```python
from build123d import *

# Parameters (mm, degrees)
EXTRUDE_1_DEPTH     = 46.5
SKETCH_4_OUTSIDE_W  = 66.66
SKETCH_4_OUTSIDE_H  = 64.16
CUT_EXTRUDE_1_DEPTH = 50
SHELL_START         = 6
SHELL_1_DEPTH       = 40.5
SHELL_START_2       = 8.5
SHELL_1_2_DEPTH     = 38
SHELL_START_3       = -22.293752824
SHELL_1_3_DEPTH     = 44.587505647
SKETCH_5_R          = 20.5
EXTRUDE_3_DEPTH     = 8
FILLET_1_R          = 5
SKETCH_4_8_R        = 3
CUT_EXTRUDE_3_DEPTH = 48
FILLET_3_R          = 3
SKETCH_8_W          = 65
SKETCH_8_H          = 50
SKETCH_8_R          = 3.25
EXTRUDE_4_DEPTH     = 8


with BuildPart() as part:
    # 草图1 → 凸台-拉伸1 (new body)
    with BuildSketch(Plane.XY):
        with BuildLine():
            ThreePointArc((35.945795724, -14), (32.1298187, -14.493507683), (28.564936874, -15.941557419))
            Line((28.564936874, -15.941557419), (25.184577361, -17.852195404))
            ThreePointArc((25.184577361, -17.852195404), (17.819425425, -19.7937446), (10.450223542, -17.867624161))
            ThreePointArc((10.450223542, -17.867624161), (0, 0), (10.450223542, 17.867624161))
            ThreePointArc((10.450223542, 17.867624161), (17.819425425, 19.7937446), (25.184577361, 17.852195404))
            Line((25.184577361, 17.852195404), (28.564936874, 15.941557419))
            ThreePointArc((28.564936874, 15.941557419), (32.1298187, 14.493507683), (35.945795724, 14))
            Line((35.945795724, 14), (49, 14))
            Line((49, 14), (49, -14))
            Line((49, -14), (35.945795724, -14))
        make_face()
    extrude(amount=EXTRUDE_1_DEPTH)

    # 草图4 outside → 切除-拉伸1 (cut, symmetric)
    with BuildSketch(Plane.XZ.offset(14)):
        with Locations((24.5, 23.25)):
            Rectangle(SKETCH_4_OUTSIDE_W, SKETCH_4_OUTSIDE_H)
        with BuildLine():
            Line((49, 36.813688531), (44, 8.5))
            Line((44, 8.5), (0, 8.5))
            Line((0, 8.5), (0, 9.114014501))
            Line((0, 9.114014501), (5, 9.114014501))
            ThreePointArc((5, 9.114014501), (9.499546785, 10.183500589), (13.036653031, 13.163198754))
            Line((13.036653031, 13.163198754), (35.472510226, 43.46311181))
            ThreePointArc((35.472510226, 43.46311181), (38.125339912, 45.697885434), (41.5, 46.5))
            Line((41.5, 46.5), (49, 46.5))
            Line((49, 46.5), (49, 36.813688531))
        make_face(mode=Mode.SUBTRACT)
    extrude(amount=CUT_EXTRUDE_1_DEPTH, both=True, mode=Mode.SUBTRACT)

    # 抽壳1: read off the stored shape, not the designer's step
    # 抽壳1 outline → 抽壳1 (add)
    with BuildSketch(Plane.XY.offset(SHELL_START)):
        with BuildLine():
            Line((49, -16.5), (49, 16.5))
            Line((49, 16.5), (35.945796372, 16.5))
            ThreePointArc((35.945796372, 16.5), (32.765815184, 16.91125632), (29.795080015, 18.117964516))
            Line((29.795080015, 18.117964516), (26.414720503, 20.028602501))
            ThreePointArc((26.414720503, 20.028602501), (17.822043244, 22.293743229), (9.224641048, 20.046602717))
            ThreePointArc((9.224641048, 20.046602717), (-2.5, 3.232e-06), (9.224641048, -20.046602717))
            ThreePointArc((9.224641048, -20.046602717), (17.822043244, -22.293743229), (26.414720503, -20.028602501))
            Line((26.414720503, -20.028602501), (29.795080015, -18.117964516))
            ThreePointArc((29.795080015, -18.117964516), (32.765815184, -16.91125632), (35.945796372, -16.5))
            Line((35.945796372, -16.5), (49, -16.5))
        make_face()
    extrude(amount=SHELL_1_DEPTH)

    # Shell 1 2 outline → Shell 1 2 (cut)
    with BuildSketch(Plane.XY.offset(SHELL_START_2)):
        with BuildLine():
            Line((25.184577361, -17.852195404), (28.564936874, -15.941557419))
            ThreePointArc((28.564936874, -15.941557419), (32.129818701, -14.493507683), (35.945795724, -14))
            Line((35.945795724, -14), (49, -14))
            Line((49, -14), (49, 14))
            Line((49, 14), (35.945795724, 14))
            ThreePointArc((35.945795724, 14), (32.129818701, 14.493507683), (28.564936874, 15.941557419))
            Line((28.564936874, 15.941557419), (25.184577361, 17.852195404))
            ThreePointArc((25.184577361, 17.852195404), (17.819425424, 19.7937446), (10.450223542, 17.867624161))
            ThreePointArc((10.450223542, 17.867624161), (0, 0), (10.450223542, -17.867624161))
            ThreePointArc((10.450223542, -17.867624161), (17.819425424, -19.7937446), (25.184577361, -17.852195404))
        make_face()
    extrude(amount=SHELL_1_2_DEPTH, mode=Mode.SUBTRACT)

    # Shell 1 3 outline → Shell 1 3 (cut)
    with BuildSketch(Plane(origin=(0, 0, 0), x_dir=(1, 0, 0), z_dir=(0, 1, 0)).offset(SHELL_START_3)):
        with BuildLine():
            Line((-4, -46.5), (41.5, -46.5))
            ThreePointArc((41.5, -46.5), (38.125339907, -45.697885432), (35.47251022, -43.463111802))
            Line((35.47251022, -43.463111802), (13.036653031, -13.163198754))
            ThreePointArc((13.036653031, -13.163198754), (9.499546673, -10.183500533), (4.999999751, -9.114014501))
            Line((4.999999751, -9.114014501), (-4, -9.114014501))
            Line((-4, -9.114014501), (-4, -46.5))
        make_face()
        Polygon((49, -36.813688531), (49, -6), (43.558517429, -6), align=None)
    extrude(amount=SHELL_1_3_DEPTH, mode=Mode.SUBTRACT)

    # 草图5 → 凸台-拉伸3 (add)
    with BuildSketch(Plane(origin=(0, 0, 6), x_dir=(-1, 0, 0), z_dir=(0, 0, -1))):
        with Locations(Location((-18, 0, 0), (0, 0, 359.999469823))):
            Circle(SKETCH_5_R)
    extrude(amount=EXTRUDE_3_DEPTH)

    # 圆角1
    fillet_1_edges = [part.edges().sort_by_distance(p)[0] for p in [
        (38.499999999, 0.000189693, -2),
    ]]
    fillet(fillet_1_edges, radius=FILLET_1_R)

    # 草图4<8> → 切除-拉伸3 (cut, symmetric)
    with BuildSketch(Plane.XZ.offset(14)):
        with Locations(Location((41.5, 39, 0), (0, 0, 270))):
            Circle(SKETCH_4_8_R)
    extrude(amount=CUT_EXTRUDE_3_DEPTH, both=True, mode=Mode.SUBTRACT)

    # 圆角3
    fillet_3_edges = [part.edges().sort_by_distance(p)[0] for p in [
        (49, -15.25, 46.5),
        (49, 15.25, 46.5),
    ]]
    fillet(fillet_3_edges, radius=FILLET_3_R)

    # 草图8 → 凸台-拉伸4 (add)
    with BuildSketch(Plane(origin=(0, 0, -2), x_dir=(-1, 0, 0), z_dir=(0, 0, -1))):
        with Locations((-18, 0)):
            Rectangle(SKETCH_8_W, SKETCH_8_H)
        with Locations((6.5, 18.846153846)):
            Circle(SKETCH_8_R, mode=Mode.SUBTRACT)
        with Locations((6.5, -18.846153846)):
            Circle(SKETCH_8_R, mode=Mode.SUBTRACT)
        with Locations((-42.5, -18.846153846)):
            Circle(SKETCH_8_R, mode=Mode.SUBTRACT)
        with Locations((-42.5, 18.846153846)):
            Circle(SKETCH_8_R, mode=Mode.SUBTRACT)
    extrude(amount=EXTRUDE_4_DEPTH)


solid = part.part
```
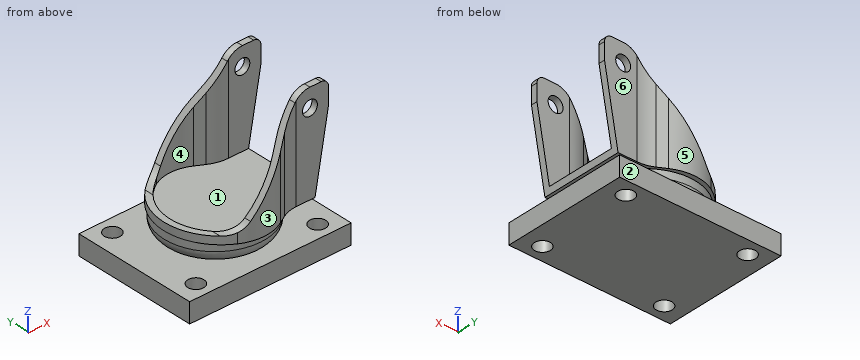
The listing builds one solid part. Answer for the finished solid, in the listing's coordinates (mm). Face numbers are marked on the shaded views. A direction names the side the tool comes from. Coordinates: 2 decimals unless noted, no trailing zeros. Loops run counter-clockwise (first coordinate to the right, second up) from the corner with the lowest first, then second, coordinate; pieces in that order, holes last. Notation, with made-up numbers: (59, 10.25) -> (79, 10.25) arc R21 cw to (79, 41.25) -> close; hole circle Ø7 at (46.25, 48). An arc over 180 degrees is marked (long way). Return JSON: item names as keys, results as strings. Group by question number.
(1) Find the intervals of material crossed by probe 1 along Y at (x, z) = (42.5, -7.75); probe 2 along Y at (x, z) = (44.5, 17); probe 3 along X at (y, z) = (20, -5.5), in increasing order. Write a range as from..to.
(2) A cutting plane is placed at A-A on x = -6.5. Write down the section's boundary in (y, z).
(3) Given pin 1 Ø14.5 at (x, z) = (40, 22) entering from +Y; pin 2 Ø12 at (x, z) = (41, 28.5) entering from -Y; pin 3 Ø2 at (y, z) = (15.5, 40.5) entering from +X; pin 4 Ø5 at (x, z) = (41.5, 39) entering from +Y, each flat-ended and moving along its own axis, determine where each tip first touches the part or whether it passes through.
(4) Which of the six approach directions +Z, -Z, +X, -X, +Y, -Y give full straight-line access (tool end or side, diameter ignored) to the marked faces 4, 5 and 6?
(5) Determine the mould class of the marked faces 1, 2 and 3 for opening direction Y: released by +Y, released by -Y, zero draft, split by the parting line, or undercut.
(6) A cutting plane is placed at B-B on z = 27. Write down the section's boundary in (x, y).
The answers:
{
 "1": {"probe 1": "y = -25..-22.1, -15.6..15.6, 22.1..25", "probe 2": "y = -16.5..-14, 14..16.5", "probe 3": "x = -14.5..-9.54, -3.46..39.46, 45.54..50.5"},
 "2": {"outline": "(-25, -10) -> (-22.1, -10) -> (-22.1, -2) -> (-25, -2) -> close; (-15.6, -10) -> (15.6, -10) -> (15.6, -2) -> (-15.6, -2) -> close; (22.1, -10) -> (25, -10) -> (25, -2) -> (22.1, -2) -> close"},
 "3": {"pin 1": "stops at y = 16.92", "pin 2": "stops at y = -16.54", "pin 3": "stops at x = 49", "pin 4": "passes through"},
 "4": {"face 4": "+Z", "face 5": "+Z, +Y", "face 6": "+Z, +X, +Y"},
 "5": {"face 1": "undercut", "face 2": "released by +Y", "face 3": "released by -Y"},
 "6": {"outline": "(23.28, -21.41) arc R17.5 ccw to (26.41, -20.03) -> (29.8, -18.12) arc R12.5 cw to (35.95, -16.5) -> (47.27, -16.5) -> (47.27, -14) -> (35.95, -14) arc R15 ccw to (28.56, -15.94) -> (25.18, -17.85) arc R15 cw to (23.28, -18.76) -> close; (23.28, 18.76) arc R15 cw to (25.18, 17.85) -> (28.56, 15.94) arc R15 ccw to (35.95, 14) -> (47.27, 14) -> (47.27, 16.5) -> (35.95, 16.5) arc R12.5 cw to (29.8, 18.12) -> (26.41, 20.03) arc R17.5 ccw to (23.28, 21.41) -> close"}
}
